Input: part model. Units: mm. Frame: model coordinates. A direction names the side the tool comes from. Coordinates: 2 decimals unless noted, no trailing zeros. Write each loop counter-clockwise with the first axis right and the second up, starting at its lowest first coordinate (ties: lowest second). Pieces come first, ordered by that corner, then holes. Notation, with made-up numbers: (70.5, 38.25) - (97.5, 38.25) arc R17 ccw to (97.5, 66.25) - close; hole circle Ø9 at (-34.5, 66). An arc over 180 degrees is marked (long way). Use a Markdown table: item, result. Add a question column.
Q1. Section query C-C (x = 3.5). Return the cut outline in (y, z), then the cut area to 3 significant figures.
Q2. Section query D-D (y = 8). Return the cut outline in (x, z), then the cut area to 3 significant figures.
Q3. Section query B-B (z = -48.65). Return the cut outline in (x, y).
Q4. Mould query, pull axis Z, two halves, no side actions, for faces 1 (the face through (-2, 0, 16)), 2 (the face through (15, 19, -40.65)), 3 (the face through (0.32, 20.14, 23.95)). Classes: released by +Z, released by -Z, zero draft, split by the parting line, or undercut.
Q5. Material intervals for probe 1 along X at (y, z) = (17.55, -48.65); probe 2 along X at (y, z) = (4, -5.5); probe 3 along X at (y, z) = (19.7, -48.65), sorted ascending. Write a range as from..to.
Q6. Set-up query: faces 4 (the face through (10.9, 20.14, -48.54)), 5 (the face through (-21, 13, -10)), 6 (the face through (17.89, 20.14, -55.75)), 7 (the face through (0, 3, 15.124)), 8 (the face through (-23, 8, -40.65)). Return all of +Z, -Z, +X, -X, +Y, -Y with unobstructed straight access to the full face (end or side cutting, diameter ignored); none if empty.
Q7. Pin query (flat end, axial travel): P1, Ø1.8, axis at x = -8, y = 3.5, coming from the -Z side; P2, Ø3, axis at x = -5, y = 18.5, coming from the -Z side; P3, Ø6, axis at x = 16, z = 12, coming from the +Y side; P4, Ø5, axis at x = -18, z = -48.65, coming from the -Y side. Return the tip coordinate at first contact, or that it passes through.
Q8. Section query A-A (z = -13). Return the cut outline in (x, y).
from build123d import *

# Parameters (mm, degrees)
SKETCH1_W           = 32
SKETCH1_H           = 30.247619048
BOSS_EXTRUDE1_DEPTH = 6
BOSS_EXTRUDE2_DEPTH = 21
BOSS_EXTRUDE3_START = 21
SKETCH1_6_R         = 3.05
BOSS_EXTRUDE3_DEPTH = 5
FILLET1_R           = 3


with BuildPart() as part:
    # Sketch1 → Boss-Extrude1 (new body)
    with BuildSketch(Plane(origin=(0, 0, 0), x_dir=(1, 0, 0), z_dir=(0, 1, 0))):
        Polygon((-26, 40.65), (-26, -24.85), (26, -24.85), (26, 40.65), (21, 40.65), (21, 19.85), (-21, 19.85), (-21, 40.65), align=None)
        Rectangle(SKETCH1_W, SKETCH1_H, mode=Mode.SUBTRACT)
    extrude(amount=BOSS_EXTRUDE1_DEPTH)

    # Sketch1_5 → Boss-Extrude2 (add)
    with BuildSketch(Plane(origin=(0, 0, 0), x_dir=(1, 0, 0), z_dir=(0, 1, 0))):
        Polygon((-26, 40.65), (-26, -24.85), (26, -24.85), (26, 40.65), (21, 40.65), (21, 19.85), (21, -19.85), (-21, -19.85), (-21, 19.85), (-21, 40.65), align=None)
    extrude(amount=BOSS_EXTRUDE2_DEPTH)

    # Sketch1_6 → Boss-Extrude3 (add)
    with BuildSketch(Plane(origin=(0, 0, 0), x_dir=(1, 0, 0), z_dir=(0, 1, 0)).offset(BOSS_EXTRUDE3_START)):
        Polygon((-26, 56.65), (-26, 40.65), (-21, 40.65), (-10, 40.65), (-10, 56.65), align=None)
        with Locations(Location((-18, 48.65, 0), (0, 0, 270))):  # turned: the seam where the file's is
            Circle(SKETCH1_6_R, mode=Mode.SUBTRACT)
        Polygon((21, 40.65), (26, 40.65), (26, 56.65), (10, 56.65), (10, 40.65), align=None)
        with Locations(Location((18, 48.65, 0), (0, 0, 270))):  # turned: the seam where the file's is
            Circle(SKETCH1_6_R, mode=Mode.SUBTRACT)
    extrude(amount=-BOSS_EXTRUDE3_DEPTH)

    # Fillet1
    fillet1_edges = [part.edges().sort_by_distance(p)[0] for p in [
        (26, 0, -7.9),
        (0, 0, 24.85),
        (-26, 0, -7.9),
        (26, 10.5, 24.85),
        (-26, 10.5, 24.85),
        (-26, 21, -15.9),
        (0, 21, 24.85),
        (26, 21, -15.9),
        (-10, 21, -48.65),
        (-18, 21, -56.65),
        (10, 21, -48.65),
        (18, 21, -56.65),
    ]]
    fillet(fillet1_edges, radius=FILLET1_R)


solid = part.part
Values follow:
| question | item | result |
|---|---|---|
| 1 | outline | (0, -19.85) - (6, -19.85) - (6, -15.12) - (0, -15.12) - close; (0, 15.12) - (6, 15.12) - (6, 19.85) - (21, 19.85) - (21, 21.85) arc R3 ccw to (18, 24.85) - (3, 24.85) arc R3 ccw to (0, 21.85) - close |
| 1 | area | 158 mm2 |
| 2 | outline | (-26, -40.65) - (-21, -40.65) - (-21, 19.85) - (21, 19.85) - (21, -40.65) - (26, -40.65) - (26, 21.85) arc R3 ccw to (23, 24.85) - (-23, 24.85) arc R3 ccw to (-26, 21.85) - close |
| 2 | area | 861 mm2 |
| 3 | outline | (-26, 16) - (-21.05, 16) - (-21.05, 21) - (-23, 21) arc R3 ccw to (-26, 18) - close; (-14.95, 16) - (-10, 16) - (-10, 18) arc R3 ccw to (-13, 21) - (-14.95, 21) - close; (10, 16) - (14.95, 16) - (14.95, 21) - (13, 21) arc R3 ccw to (10, 18) - close; (21.05, 16) - (26, 16) - (26, 18) arc R3 ccw to (23, 21) - (21.05, 21) - close |
| 4 | face 1 | zero draft |
| 4 | face 2 | undercut |
| 4 | face 3 | released by +Z |
| 5 | probe 1 | -26..-21.05, -14.95..-10, 10..14.95, 21.05..26 |
| 5 | probe 2 | -26..-16, 16..26 |
| 5 | probe 3 | -25.47..-21.05, -14.95..-10.53, 10.53..14.95, 21.05..25.47 |
| 6 | face 4 | -Z, +Y |
| 6 | face 5 | +Y |
| 6 | face 6 | -Z, +X, -X, +Y |
| 6 | face 7 | +Y, -Y |
| 6 | face 8 | -Z, +X, -X, -Y |
| 7 | P1 | z = -19.85 |
| 7 | P2 | z = 19.85 |
| 7 | P3 | y = 6 |
| 7 | P4 | through |
| 8 | outline | (-26, 3) arc R3 ccw to (-23, 0) - (-16, 0) - (-16, 6) - (-21, 6) - (-21, 21) - (-23, 21) arc R3 ccw to (-26, 18) - close; (16, 0) - (23, 0) arc R3 ccw to (26, 3) - (26, 18) arc R3 ccw to (23, 21) - (21, 21) - (21, 6) - (16, 6) - close |
